Source: CAD feature listing. Evaluate the final solid. Frame: model axes, mm. A direction names the side the tool comes from. Round coordinates to 2 decimals unless told otherwise and drop trailing zeros. Order: outer loops, then holes, each group sorted by start corner. A loop starts at its lowest first (then second) coordinate and runs counter-clockwise, first axis right, second up. Notation, with made-up numbers: (33, 3.25) -> (41, 3.25) arc R20 ccw to (41, 8.25) -> close; hole circle Ø8 at (0, 17.25). An arc over 180 degrees is marked (long way). Answer as CSV lines item,"result". Start each with the question number.
(1) Section query B-B (y = 6). Output: boundary loops of the cut face in (x, z), plus the area to 3 significant figures.
(2) Section query C-C (z = -3.5). Output: boundary loops of the cut face in (x, y).
(3) Set-up query: faces 1 (the cylindrical face through (27.614, 5.144, -4.782)), 2 (the flat face through (1, 0, -7)), 3 (the flat face through (9, 11.25, -8)), 4 (the flat face through (9, 6, 0)), 5 (the flat face through (9, 0.75, -8)). Return all of +Z, -Z, +X, -X, +Y, -Y with unobstructed straight access to the full face (end or side cutting, diameter ignored); none if empty.
(4) Line query: line 1 along X through (y, z) = (11.75, -13); line 2 along X through (y, z) = (6, -7.2); line 3 along Y through (x, z) = (35.7, -7.6). Output: solid intervals per line, ascending. Write a range as from..to.
(5) Contact query for flat-ended pins moving along their axis: P1, Ø0.8, axis at y = 0, z = -8, coming from the +X side; P2, Ø1.9, axis at x = 35.7, y = 6, coming from the +Z side; P3, Ø5, axis at x = 32, z = -12.5, coming from the -Y side. Output: stop coordinate, or through.
(6) Section query D-D (x = 22). Output: boundary loops of the cut face in (y, z).
(7) Pull-direction query (X, two-part tool) for faces 6 (the cylindrical face through (35.1, 6, -7.5)), 7 (the flat face through (18, 9, -6)), 8 (the flat face through (9, 6, -15)); classes: +X half, -X half, draft (parallel to the pull), parting line (faces both ways), or undercut.
(8) Section query A-A (z = -7.5). Output: boundary loops of the cut face in (x, y).
```python
from build123d import *

# Parameters (mm, degrees)
SKETCH1_W               = 10
SKETCH1_H               = 8
BOSS_EXTRUDE5_DEPTH     = 12
SKETCH2_R               = 1.9
BOSS_EXTRUDE6_DEPTH     = 13
CUT_EXTRUDE1_DEPTH      = 3
CUT_EXTRUDE1_DEPTH_BACK = 3
SKETCH3_R               = 0.4
SKETCH4_W               = 10
SKETCH4_H               = 0.5
CUT_EXTRUDE2_DEPTH      = 10
SCALE1_SCALE            = 1.5


with BuildPart() as part:
    # Sketch1 → Boss-Extrude5 (new body)
    with BuildSketch(Plane(origin=(0, 0, 0), x_dir=(0, 0, -1), z_dir=(1, 0, 0))):
        with Locations((5, 4)):
            Rectangle(SKETCH1_W, SKETCH1_H)
    extrude(amount=BOSS_EXTRUDE5_DEPTH)

    # Sketch2 → Boss-Extrude6 (add)
    with BuildSketch(Plane(origin=(12, 0, 0), x_dir=(0, 0, -1), z_dir=(1, 0, 0))):
        with Locations(Location((5, 4, 0), (0, 0, 180))):
            Circle(SKETCH2_R)
    extrude(amount=BOSS_EXTRUDE6_DEPTH)

    # Sketch3 → Cut-Extrude1 (cut, two sides: drawn at the far end of the back side and taken through both)
    with BuildSketch(Plane(origin=(0, 0, -5), x_dir=(-1, 0, 0), z_dir=(0, 0, -1)).offset(-CUT_EXTRUDE1_DEPTH_BACK)):
        with Locations(Location((-23.8, 4, 0), (0, 0, 180))):
            Circle(SKETCH3_R)
    extrude(amount=CUT_EXTRUDE1_DEPTH + CUT_EXTRUDE1_DEPTH_BACK, mode=Mode.SUBTRACT)

    # Sketch4 → Cut-Extrude2 (cut)
    with BuildSketch(Plane(origin=(0, 0, -10), x_dir=(-1, 0, 0), z_dir=(0, 0, -1))):
        with Locations((-6, 7.75)):
            Rectangle(SKETCH4_W, SKETCH4_H)
        with Locations((-6, 0.25)):
            Rectangle(SKETCH4_W, SKETCH4_H)
    extrude(amount=-CUT_EXTRUDE2_DEPTH, mode=Mode.SUBTRACT)


with BuildPart() as part_1:
    # Scale1: scaled about (0, 0, 0)
    add(part.part.scale(SCALE1_SCALE))


solid = part_1.part
```
Answer block:
1,outline,"(0, -15) -> (18, -15) -> (18, -10.35) -> (35.1, -10.35) -> (35.1, -4.65) -> (18, -4.65) -> (18, 0) -> (0, 0) -> close; (36.3, -10.35) -> (37.5, -10.35) -> (37.5, -4.65) -> (36.3, -4.65) -> close"
1,area,"374 mm2"
2,outline,"(0, 0) -> (1.5, 0) -> (1.5, 0.75) -> (16.5, 0.75) -> (16.5, 0) -> (18, 0) -> (18, 12) -> (16.5, 12) -> (16.5, 11.25) -> (1.5, 11.25) -> (1.5, 12) -> (0, 12) -> close"
3,face 1,"+X"
3,face 2,"+Z, -Z, +X, -X, -Y"
3,face 3,"+Z, -Z, +Y"
3,face 4,"+Z, +X, -X, +Y, -Y"
3,face 5,"+Z, -Z, -Y"
4,line 1,"0..1.5, 16.5..18"
4,line 2,"0..35.1, 36.3..37.5"
4,line 3,"3.15..5.4, 6.6..8.85"
5,P1,"x = 18"
5,P2,"z = -4.65"
5,P3,"y = 4.63"
6,outline,"circle Ø5.7 at (6, -7.5)"
7,face 6,"undercut"
7,face 7,"+X half"
7,face 8,"draft"
8,outline,"(0, 0) -> (1.5, 0) -> (1.5, 0.75) -> (16.5, 0.75) -> (16.5, 0) -> (18, 0) -> (18, 3.15) -> (37.5, 3.15) -> (37.5, 8.85) -> (18, 8.85) -> (18, 12) -> (16.5, 12) -> (16.5, 11.25) -> (1.5, 11.25) -> (1.5, 12) -> (0, 12) -> close; hole circle Ø1.2 at (35.7, 6)"
